Verification items for this drawing (mm, ordinates from the low corner). A direction names the side the tool comes from. Coordinates: 2 decimals unless noted, no trailing zeros. Order: outer loops, then holes, each group sorted by start corner. A loop starts at its lowest first (then second) coordinate and runs counter-clockwise, first axis right, second up. Notation, with made-up numbers: M -29,26.5 L 11,26.5 A13 cw 11,44.5 Z; hole C 38,-33 d8. An arc over 180 degrees is marked long. Return JSON: item names as keys, results as strings. Group by question number.
1. Mould release check, pull along X, two halves, no side actions. Record for the marked faces 1, 2, 3 and 4: +X half, -X half, draft (parallel to the pull), parting line (faces both ways), or undercut.
2. Set-up check for the marked faces 5 and 6: record each of +Z, -Z, +X, -X, +Y, -Y from which the full face is reachable in a straight line by a thin tool's end or side.
3. Section check C-C, the plane z = 76. Record the cut outline in (x, y), plus the area to 3 significant figures.
4. Section check D-D, the plane z = 21. Record the cut outline in (x, y).
5. Section check B-B, the plane y = 17.5. Record the cut outline in (x, z), plus the area to 3 significant figures.
6. Material ranges on line 1 along X through (y, z) = (12.5, 33); line 2 along X through (y, z) = (13, 12), recorded low to high.
7. Section check A-A, the plane x = 11. Record the cut outline in (y, z), plus the area to 3 significant figures.
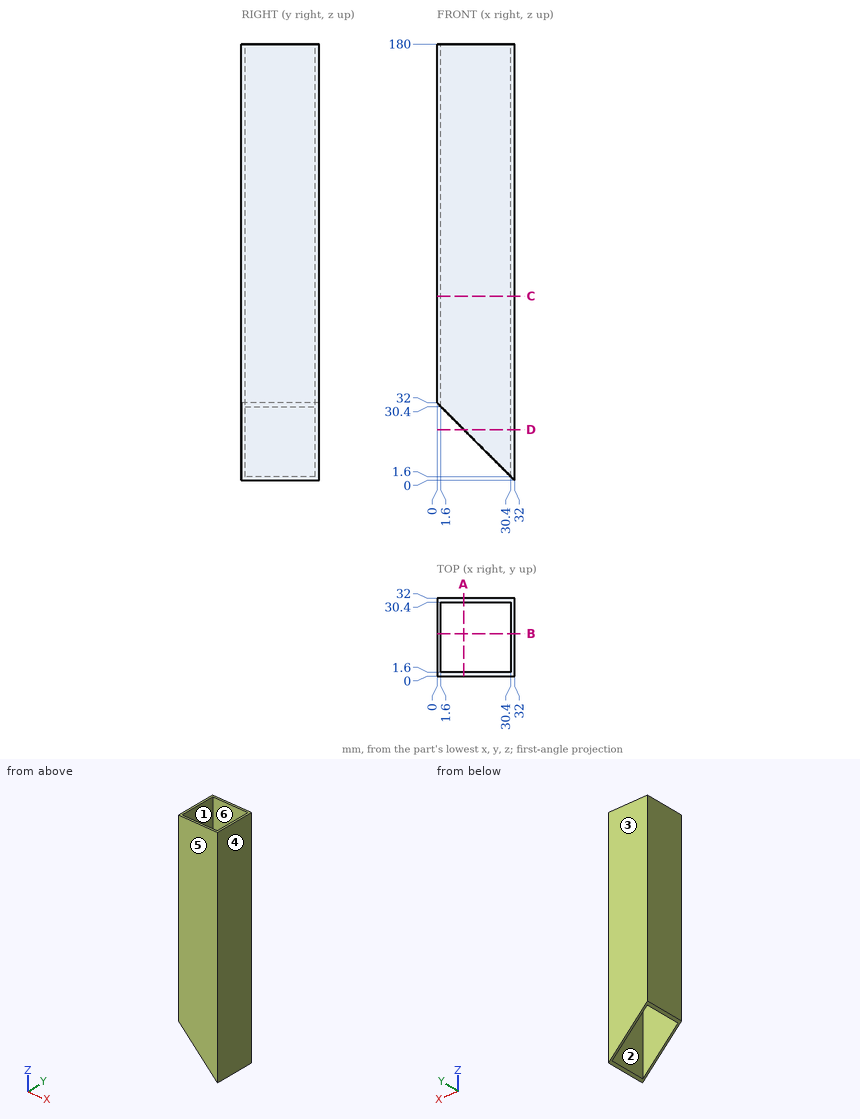
Answers follow:
{
 "1": {"face 1": "undercut", "face 2": "undercut", "face 3": "draft", "face 4": "+X half"},
 "2": {"face 5": "+Z, -Z, +X, -X, -Y", "face 6": "+Z, -Z"},
 "3": {"outline": "M 0,0 L 32,0 L 32,32 L 0,32 Z; hole M 1.6,1.6 L 30.4,1.6 L 30.4,30.4 L 1.6,30.4 Z", "area": "195 mm^2"},
 "4": {"outline": "M 11,0 L 32,0 L 32,32 L 11,32 L 11,30.4 L 30.4,30.4 L 30.4,1.6 L 11,1.6 Z"},
 "5": {"outline": "M 0,32 L 1.6,30.4 L 1.6,180 L 0,180 Z; M 30.4,1.6 L 32,0 L 32,180 L 30.4,180 Z", "area": "525 mm^2"},
 "6": {"line 1": "0 to 1.6, 30.4 to 32", "line 2": "30.4 to 32"},
 "7": {"outline": "M 0,21 L 1.6,21 L 1.6,180 L 0,180 Z; M 30.4,21 L 32,21 L 32,180 L 30.4,180 Z", "area": "509 mm^2"}
}
